Autodesk Inventor part; units mm, degrees
ref_plane "YZ Plane" through (0, 0, 0) normal (1, 0, 0) x (0, 1, 0)
ref_plane "XZ Plane" through (0, 0, 0) normal (0, 1, 0) x (-1, 0, 0)
ref_plane "XY Plane" through (0, 0, 0) normal (0, 0, 1) x (1, 0, 0)
sketch "Sketch1" plane through (0, 0, 0) normal (0, 1, 0) x (-1, 0, 0)
  line L0 (0, -7.3406) -> (-6.3571, -3.6703)
  line L1 (-6.3571, -3.6703) -> (-6.3571, 3.6703)
  line L2 (-6.3571, 3.6703) -> (0, 7.3406)
  line L3 (0, 7.3406) -> (6.3571, 3.6703)
  line L4 (6.3571, 3.6703) -> (6.3571, -3.6703)
  line L5 (6.3571, -3.6703) -> (0, -7.3406)
  point P0 (0, 0)
  point P1 (0, 0)
  dimension "d0" = 7.3406
extrude "Extrusion1" add sketch "Sketch1" along normal blind 50.8
properties part number "Arm short hex"
Check sheet for the modelled part. Datum: model origin and axes. Units: mm. Round coordinates to 2 decimals unless told otherwise and drop trailing zeros. Loops run counter-clockwise (first coordinate to the right, second up) from the corner with the lowest first, then second, coordinate; pieces in that order, holes last.
1. Sectioned sample at B-B on x = 5. Record the boundary of the cut face in (y, z).
2. Gauge pin test, flat ends, axial feed: pin 1 Ø4 at (x, y) = (-3, 38) entering from +Z; pin 2 Ø5 at (x, y) = (0.5, 31) entering from -Z; pin 3 Ø4 at (x, y) = (-4, 32) entering from -Z. Record the tip position at first contact, or that the pin passes through.
3. Sectioned sample at C-C on z = -4.75. Record the boundary of the cut face in (x, y).
4. Scan lines: probe 1 along X at (y, z) = (48.5, 4.75); probe 2 along Z at (x, y) = (4.25, 23.5); probe 3 along X at (y, z) = (47, 6.5). Record each from-to range of solid material in increasing order.
5. Sectioned sample at A-A on y = 21.5. Record the boundary of the cut face in (x, z), and give its area (3 significant figures).
Recorded:
1. outline: (0, -4.45) - (50.8, -4.45) - (50.8, 4.45) - (0, 4.45) - close
2. pin 1: stops at z = 6.76
2. pin 2: stops at z = -7.34
2. pin 3: stops at z = -6.19
3. outline: (-4.49, 0) - (4.49, 0) - (4.49, 50.8) - (-4.49, 50.8) - close
4. probe 1: x = -4.49 to 4.49
4. probe 2: z = -4.89 to 4.89
4. probe 3: x = -1.46 to 1.46
5. outline: (-6.36, -3.67) - (0, -7.34) - (6.36, -3.67) - (6.36, 3.67) - (0, 7.34) - (-6.36, 3.67) - close
5. area: 140 mm2
